Part model, mm, in its own coordinate system. A direction names the side the tool comes from. Coordinates: 2 decimals unless noted, no trailing zeros. Write each loop counter-clockwise with the first axis right and the second up, starting at its lowest first coordinate (ties: lowest second). Pieces come first, ordered by that corner, then holes. Notation, with made-up numbers: (31.25, -8.5) -> (82.25, -8.5) arc R21 ccw to (82.25, 2.5) -> close; hole circle Ø4 at (27.5, 88). An arc over 180 degrees is marked (long way). Write item = value, one per line. Start each with the question number.
Q1. Pull direction X, two halves, no side cores. Call faces 1 (the cylindrical face through (-5, -13, 12)), 2 (the cylindrical face through (4, 14, 12)), 3 (the flat face through (0, -15, 12)), 4 (the flat face through (0, 0, 10)): released by +X, released by -X, zero draft, split by the parting line, or undercut.
Q2. Probe line 1 (Y direction, x = 0, z = 11.45); line 2 (Y direction, x = -4, z = 6); line 3 (Z direction, x = -2.25, y = 7). List the from-to ranges inside material, lowest first.
Q3. Pin check, flat tips, straight feed: P1, Ø1.5, axis at x = -3, y = 9.5, coming from the -Z side; P2, Ø1, axis at y = -2, z = 8.5, coming from the +X side; P3, Ø3.5, axis at x = -1, y = -5.5, coming from the -Z side. Stop position of each tip, or through.
Q4. Band-saw the part on A-A, the plane x = 0. List the corners of the cut face in (y, z).
Q5. Band-saw the part on B-B, the plane y = 0. List the corners of the cut face in (x, z), plus the area to 3 significant figures.
Q6. Band-saw the part on C-C, the plane z = 12.25. List the corners of the cut face in (x, y), plus the area to 3 significant figures.
Q7. Band-saw the part on D-D, the plane z = 6. List the corners of the cut face in (x, y).
Q8. Tool access for faces 5 (the cylindrical face through (-0.54, -2.44, 4.93)), 6 (the flat face through (6, 0, 12)): list every direction of +Z, -Z, +X, -X, +Y, -Y with a clear straight run to the whole face (end or side of a thin tool).
from build123d import *

# Parameters (mm, degrees)
F0_R     = 5
F0_R_2   = 2.5
F1_DEPTH = 10
F2_W     = 12
F2_H     = 30
F2_R     = 1.5
F3_DEPTH = 3.5
F4_R     = 5
F5_R     = 2


with BuildPart() as f1:
    # F0 (on Top) → F1 (new body)
    with BuildSketch(Plane.XY):
        Circle(F0_R)
        Circle(F0_R_2, mode=Mode.SUBTRACT)
    extrude(amount=F1_DEPTH)

    # F2 (on face) → F3 (join)
    with BuildSketch(Plane.XY.offset(10)):
        Rectangle(F2_W, F2_H)
        with Locations((0, -10)):
            Circle(F2_R, mode=Mode.SUBTRACT)
        with Locations((0, 10)):
            Circle(F2_R, mode=Mode.SUBTRACT)
    extrude(amount=F3_DEPTH)

    # F4
    f4_edges = [f1.edges().sort_by_distance(p)[0] for p in [
        (6, 15, 11.75),
        (-6, 15, 11.75),
        (-6, -15, 11.75),
        (6, -15, 11.75),
    ]]
    fillet(f4_edges, radius=F4_R)

    # F5
    f5_edges = [f1.edges().sort_by_distance(p)[0] for p in [
        (-5, 0, 0),
    ]]
    fillet(f5_edges, radius=F5_R)


solid = f1.part
Ans:
q1.face_1 = released by -X
q1.face_2 = released by +X
q1.face_3 = zero draft
q1.face_4 = undercut
q2.line_1 = -15 to -11.5, -8.5 to 8.5, 11.5 to 15
q2.line_2 = -3 to 3
q2.line_3 = 10 to 13.5
q3.P1 = 10
q3.P2 = 4.77
q3.P3 = 0.19
q4.outline = (-15, 10) -> (-11.5, 10) -> (-11.5, 13.5) -> (-15, 13.5) -> close; (-8.5, 10) -> (-5, 10) -> (-5, 2) arc R2 ccw to (-3, 0) -> (-2.5, 0) -> (-2.5, 10) -> (2.5, 10) -> (2.5, 0) -> (3, 0) arc R2 ccw to (5, 2) -> (5, 10) -> (8.5, 10) -> (8.5, 13.5) -> (-8.5, 13.5) -> close; (11.5, 10) -> (15, 10) -> (15, 13.5) -> (11.5, 13.5) -> close
q5.outline = (-6, 10) -> (-5, 10) -> (-5, 2) arc R2 ccw to (-3, 0) -> (-2.5, 0) -> (-2.5, 10) -> (2.5, 10) -> (2.5, 0) -> (3, 0) arc R2 ccw to (5, 2) -> (5, 10) -> (6, 10) -> (6, 13.5) -> (-6, 13.5) -> close
q5.area = 90.3 mm2
q6.outline = (-6, -10) arc R5 ccw to (-1, -15) -> (1, -15) arc R5 ccw to (6, -10) -> (6, 10) arc R5 ccw to (1, 15) -> (-1, 15) arc R5 ccw to (-6, 10) -> close; hole circle Ø3 at (0, -10); hole circle Ø3 at (0, 10)
q6.area = 324 mm2
q7.outline = circle Ø10 at (0, 0); hole circle Ø5 at (0, 0)
q8.face_5 = -Z
q8.face_6 = +Z, -Z, +X, +Y, -Y
